Model file for the job. Use its own axes, mm. Face numbers are marked on the shaded views. A direction names the side the tool comes from. Coordinates: 2 decimals unless noted, no trailing zeros. Order: outer loops, then holes, each group sorted by start corner. A loop starts at its lowest first (then second) coordinate and runs counter-clockwise, first axis right, second up.
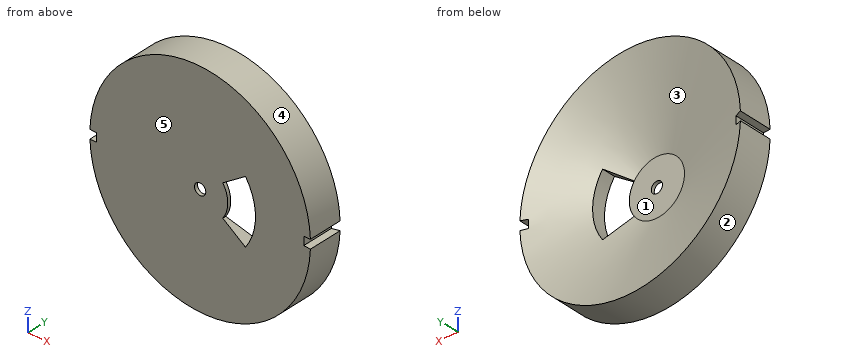
Autodesk Inventor part; units mm, degrees
ref_plane "YZ Plane" through (0, 0, 0) normal (1, 0, 0) x (0, 1, 0)
ref_plane "XZ Plane" through (0, 0, 0) normal (0, 1, 0) x (-1, 0, 0)
ref_plane "XY Plane" through (0, 0, 0) normal (0, 0, 1) x (1, 0, 0)
sketch "Sketch2" plane through (0, 0, 0) normal (0, 0, 1) x (1, 0, 0)
  line L0 (-50, 0) -> (-99.9, 0)
  line L1 (-99.9, 0) -> (-99.9, 30)
  line L2 (0, 0) -> (0, 50.0549)
  line L3 (-99.9, 30) -> (-25, 3)
  line L4 (-50, 0) -> (0, 0)
  line L5 (-25, 3) -> (0, 3)
  line L6 (0, 3) -> (0, 0)
  point P0 (-99.9, 15)
  dimension "d2" = 30
  dimension "d6" = 199.8
  dimension "d15" = 50
  dimension "d16" = 3
revolve "Revolution1" add sketch "Sketch2" angle 360 about axis through (0, 0, 0) along (0, 1, 0)
sketch "Sketch3" plane through (0, 0, 0) normal (0, -1, 0) x (1, 0, 0)
  circle A0 centre (0, 0) radius 99.9
  line L0 (0, 0) -> (99.8199, 4)
  line L1 (0, 0) -> (99.8199, -4)
  line L2 (0, 0) -> (99.9, 0) construction
  line L3 (11.4718, 0) -> (11.4718, -0.4597) construction
  line L4 (11.4718, 0) -> (11.4718, 0.4597) construction
  circle A1 centre (0, 0) radius 93.9
  point P0 (93.8247, 3.7598)
  point P1 (93.8247, -3.7598)
  dimension "d8" = 8
  dimension "d9" = 6
extrude "Extrusion1" cut sketch "Sketch3" against normal through all contours A0 L1 A1 L0 picked at (97.8363, 3.4756)
pattern_circular "Circular Pattern1" count 2 over 360 about axis through (0, 16.5, 0) along (0, 1, 0) of "Extrusion1"
sketch "Sketch5" plane through (0, 3, 0) normal (0, 1, 0) x (1, 0, 0)
  point P0 (0, 0)
  point P1 (0, 0)
hole "Hole1" at (0, 3, 0) direction (0, -1, 0) diameter 10.2 end through all
sketch "Sketch6" plane through (0, 0, 0) normal (0, -1, 0) x (1, 0, 0)
  line L0 (0, 0) -> (93.9, 0) construction
  arc A0 (93.8247, -3.7598) -> (93.8247, 3.7598) centre (0, 0) ccw
  arc A1 (41.0395, -28.7362) -> (41.0395, 28.7362) centre (0, 0) ccw
  line L1 (0, 0) -> (41.0395, 28.7362)
  line L2 (0, 0) -> (41.0395, -28.7362)
  line L3 (16.9605, 0) -> (16.9605, 11.8759) construction
  line L4 (16.9605, 0) -> (16.9605, -11.8759) construction
  arc A2 (20.4788, -14.3394) -> (20.4788, 14.3394) centre (0, 0) ccw
  point P0 (25, 0)
  dimension "d30" = 50.1
  dimension "d31" = 70
  dimension "d32" = 25
extrude "Extrusion3" cut sketch "Sketch6" against normal through all contours L2 A2 L1 A1
properties part number "feeder"
Q1. Probe line 1 (X direction, y = 0.8, z = 0); line 2 (Z direction, x = 0, y = 1.9); line 3 (Z direction, x = 36.5, y = 9.5). List the from-to ranges inside material, lowest first.
Established:
line 1: x = -93.9 to -5.1, 5.1 to 25, 50.1 to 93.9
line 2: z = -99.9 to -5.1, 5.1 to 99.9
line 3: z = -92.99 to -25.56, 25.56 to 92.99
Q2. Which spindle directions (+Z, -Z, +X, -X, +Y, -Y) get a long thin tool onto all of the face, cutting with end or side? Do the marked faces 1 and 2. Say none if no direction does.
Established:
face 1: +Y
face 2: -Z, +Y, -Y
Q3. Cut at A-A, the plane x = 0. List the corners of the cut face in (y, z), plus the area to 3 significant figures.
Established:
outline: (0, -99.9) - (30, -99.9) - (3, -25) - (3, -5.1) - (0, -5.1) - close; (0, 5.1) - (3, 5.1) - (3, 25) - (30, 99.9) - (0, 99.9) - close
area: 2,590 mm2
Q4. Drop flat-ended pins along their axis: P1, Ø8, axis at y = 9, z = 26.5, coming from the -X side; P2, Ø6, axis at y = 16, z = -73, coming from the +X side; P3, Ø4, axis at x = -24, y = 21, coming from the -Z side; P4, Ø9, axis at x = 0, z = 0, coming from the -Y side. Give the stop position or say it passes through.
Established:
P1: stops at x = -97.33
P2: stops at x = 71.27
P3: stops at z = -97.45
P4: passes through
Q5. Cut at C-C, the plane y = 23. List the corners of the cut face in (x, z), plus the area to 3 significant figures.
Established:
outline: (-99.82, -4) arc R99.9 ccw to (99.82, -4) - (93.82, -3.76) arc R93.9 ccw to (93.82, 3.76) - (99.82, 4) arc R99.9 ccw to (-99.82, 4) - (-93.82, 3.76) arc R93.9 ccw to (-93.82, -3.76) - close; hole circle Ø160.96 at (0, 0)
area: 10,900 mm2
Q6. Mould opens along X. For the marked faces 3, 4 and 5 say: pulls with the +X half, pulls with the -X half, needs draft (parallel to the pull), parting line crosses it, or undercut.
Established:
face 3: undercut
face 4: parting line crosses it
face 5: needs draft
Q7. Cut at B-B, the plane z = 0. List the corners of the cut face in (x, y).
Established:
outline: (-93.9, 0) - (-5.1, 0) - (-5.1, 3) - (-25, 3) - (-93.9, 27.84) - close; (5.1, 0) - (25, 0) - (25, 3) - (5.1, 3) - close; (50.1, 0) - (93.9, 0) - (93.9, 27.84) - (50.1, 12.05) - close
